from build123d import *

# Parameters (mm, degrees)
SKETCH023_W     = 340
SKETCH023_H     = 384
SKETCH023_R     = 1.7
SKETCH023_R_2   = 6.5
SKETCH023_R_3   = 10
PAD015_DEPTH    = 8
SKETCH040_W     = 340
SKETCH040_H     = 8.1
POCKET009_DEPTH = 4.1


with BuildPart() as wall_inner:
    # Sketch023 → Pad015 (new body)
    with BuildSketch(Plane.XY.offset(40)):
        with Locations((210, 0)):
            Rectangle(SKETCH023_W, SKETCH023_H)
        with Locations((226.376606, 58.25)):
            Circle(SKETCH023_R, mode=Mode.SUBTRACT)
        with Locations((253.223394, 58.25)):
            Circle(SKETCH023_R, mode=Mode.SUBTRACT)
        with Locations((239.8, 35)):
            Circle(SKETCH023_R, mode=Mode.SUBTRACT)
        with Locations((246.8, 50.5)):
            Circle(SKETCH023_R_2, mode=Mode.SUBTRACT)
        with Locations((70, 180)):
            Circle(SKETCH023_R_3, mode=Mode.SUBTRACT)
        with Locations((330, 180)):
            Circle(SKETCH023_R_3, mode=Mode.SUBTRACT)
        with Locations((70, -180)):
            Circle(SKETCH023_R_3, mode=Mode.SUBTRACT)
        with Locations((330, -180)):
            Circle(SKETCH023_R_3, mode=Mode.SUBTRACT)
    extrude(amount=-PAD015_DEPTH)

    # Sketch040 → Pocket009 (cut)
    with BuildSketch(Plane.XY.offset(40)):
        with Locations((210, 164.05)):
            Rectangle(SKETCH040_W, SKETCH040_H)
        with Locations((210, -164.05)):
            Rectangle(SKETCH040_W, SKETCH040_H)
    extrude(amount=-POCKET009_DEPTH, mode=Mode.SUBTRACT)


with BuildPart() as part_mirroring004:
    # Part__Mirroring004: instance of Wall-inner
    add(wall_inner.part.mirror(Plane(origin=(0, 0, 200), x_dir=(0, 1, 0), z_dir=(0, 0, 1))))


solid = part_mirroring004.part
Geometry: final body of the model. Coordinates: model frame, mm. A direction names the side the tool comes from. Coordinates: 2 decimals unless noted, no trailing zeros. Order: outer loops, then holes, each group sorted by start corner. A loop starts at its lowest first (then second) coordinate and runs counter-clockwise, first axis right, second up.
1) Ray query, probe 1 along Y at (x, z) = (246.8, 363); probe 2 along Y at (x, z) = (141.5, 363); probe 3 along Y at (x, z) = (330, 364.75). Return the intervals inside material, ascending.
Result sheet:
probe 1: y = -192 to -168.1, -160 to 44, 57 to 160, 168.1 to 192
probe 2: y = -192 to -168.1, -160 to 160, 168.1 to 192
probe 3: y = -192 to -190, -170 to 170, 190 to 192
2) Section B-B (y = 50.5). Return loops of the section in (x, z).
Result sheet:
outline: (40, 360) - (240.3, 360) - (240.3, 368) - (40, 368) - close; (253.3, 360) - (380, 360) - (380, 368) - (253.3, 368) - close
3) Section C-C (z = 362.25). Give the number of separate pieces and of enclosed holes in the cut face, then the cut area to 3 significant figures.
Result sheet:
separate pieces: 3
enclosed holes: 8
area: 124,000 mm2
4) Draft query along Y for faces 3 (the flat face through (208, 180, 360)), 4 (the flat face through (208, -192, 364)), 5 (the flat face through (208, 192, 364)), 6 (the cylindrical face through (322, 174, 364)). Return one class per face: released by +Y, released by -Y, zero draft, split by the parting line, or undercut.
Result sheet:
face 3: zero draft
face 4: released by -Y
face 5: released by +Y
face 6: undercut
5) Section A-A (x = 246.8). Return loops of the section in (y, z), then the cut area to 3 significant figures.
Result sheet:
outline: (-192, 360) - (-168.1, 360) - (-168.1, 364.1) - (-160, 364.1) - (-160, 360) - (44, 360) - (44, 368) - (-192, 368) - close; (57, 360) - (160, 360) - (160, 364.1) - (168.1, 364.1) - (168.1, 360) - (192, 360) - (192, 368) - (57, 368) - close
area: 2,900 mm2
6) First-contact query: P1, Ø2, axis at x = 253.22, y = 58.25, coming from the -Z side; P2, Ø2.5, axis at x = 261, y = -163, coming from the -Z side; P3, Ø4.5, axis at x = 239.8, y = 35, coming from the +Z side. Flat tips, straight axial feed; report the tip coordinate or a pass-through.
Result sheet:
P1: passes through
P2: stops at z = 364.1
P3: stops at z = 368
7) Section D-D (x = 330). Return loops of the section in (y, z), then the cut area to 3 significant figures.
Result sheet:
outline: (-192, 360) - (-190, 360) - (-190, 368) - (-192, 368) - close; (-170, 360) - (-168.1, 360) - (-168.1, 364.1) - (-160, 364.1) - (-160, 360) - (160, 360) - (160, 364.1) - (168.1, 364.1) - (168.1, 360) - (170, 360) - (170, 368) - (-170, 368) - close; (190, 360) - (192, 360) - (192, 368) - (190, 368) - close
area: 2,690 mm2
8) Set-up query: faces 1 (the cylindrical face through (322, -186, 364)), 2 (the flat face through (208, 164, 364.1)). Return all of +Z, -Z, +X, -X, +Y, -Y with unobstructed straight access to the full face (end or side cutting, diameter ignored); none if empty.
Result sheet:
face 1: +Z, -Z
face 2: -Z, +X, -X
